Geometry check sheet. Reference: the model listing, model coordinates, mm. A direction names the side the tool comes from. Give positions to 0.01 mm unless a question says otherwise; leave off trailing zeros. Loops run counter-clockwise (first coordinate to the right, second up) from the corner with the lowest first, then second, coordinate; pieces in that order, holes last. Notation, with made-up numbers: (-22, 7) -> (-5, 7) arc R23 cw to (-5, 43) -> close; hole circle Ø9 at (26.5, 78). An arc over 180 degrees is marked (long way). Write item = value, one per line.
```python
from build123d import *

# Parameters (mm, degrees)
SKETCH1_W                                  = 120.9294
SKETCH1_H                                  = 116.1796
SKETCH1_R                                  = 10.5
SKETCH1_W_2                                = 11.906
SKETCH1_H_2                                = 30.0122
SKETCH1_W_3                                = 76.19975
SKETCH1_H_3                                = 95.2627
BOSS_EXTRUDE1_DEPTH                        = 4
SKETCH2_W                                  = 116.1796
SKETCH2_H                                  = 120.9294
SKETCH2_W_2                                = 102.459137156
SKETCH2_H_2                                = 106.648
BOSS_EXTRUDE2_DEPTH                        = 4.75
CUT_EXTRUDE1_DEPTH                         = 1.25
SKETCH6_W                                  = 25.4
SKETCH6_H                                  = 2.0635
SKETCH6_W_2                                = 1.783031422
SKETCH6_H_2                                = 25.4
CUT_EXTRUDE2_DEPTH                         = 2
CUT_EXTRUDE3_DEPTH                         = 10.16
SKETCH8_R                                  = 1.3
CUT_EXTRUDE4_DEPTH                         = 4
MIRROR1_AT_THE_SECOND_PLANE_COPY_1_SKETC_R = 1.3
MIRROR1_AT_THE_SECOND_PLANE_COPY_1_DEPTH   = 4
FILLET1_R                                  = 5
CHAMFER1_SIZE                              = 4


with BuildPart() as part:
    # Sketch1 → Boss-Extrude1 (new body)
    with BuildSketch(Plane(origin=(0, 0, 0), x_dir=(0, 1, 0), z_dir=(0, 0, 1))):
        Rectangle(SKETCH1_W, SKETCH1_H)
        with Locations(Location((39.3375, 10.8746, 0), (0, 0, 270))):
            Circle(SKETCH1_R, mode=Mode.SUBTRACT)
        with Locations((39.2905, -23.9125)):
            Rectangle(SKETCH1_W_2, SKETCH1_H_2, mode=Mode.SUBTRACT)
        with Locations((-11.906375, 0)):
            Rectangle(SKETCH1_W_3, SKETCH1_H_3, mode=Mode.SUBTRACT)
    extrude(amount=BOSS_EXTRUDE1_DEPTH)

    # Sketch2 → Boss-Extrude2 (add)
    with BuildSketch(Plane(origin=(0, 0, 0), x_dir=(-1, 0, 0), z_dir=(0, 0, -1))):
        Rectangle(SKETCH2_W, SKETCH2_H)
        Rectangle(SKETCH2_W_2, SKETCH2_H_2, mode=Mode.SUBTRACT)
    extrude(amount=BOSS_EXTRUDE2_DEPTH)

    # Sketch4 → Cut-Extrude1 (cut)
    with BuildSketch(Plane(origin=(0, 0, -4.75), x_dir=(-1, 0, 0), z_dir=(0, 0, -1))):
        Polygon((-50.0126, -52.3875), (-21, -52.3875), (-16, -57.3875), (16, -57.3875), (21, -52.3875), (50.0126, -52.3875), (50.0126, -21), (55.0126, -16), (55.0126, 16), (50.0126, 21), (50.0126, 52.3875), (21, 52.3875), (16, 57.3875), (-16, 57.3875), (-21, 52.3875), (-50.0126, 52.3875), (-50.0126, 21), (-55.0126, 16), (-55.0126, -16), (-50.0126, -21), align=None)
    extrude(amount=-CUT_EXTRUDE1_DEPTH, mode=Mode.SUBTRACT)

    # Sketch6 → Cut-Extrude2 (cut)
    with BuildSketch(Plane(origin=(0, 0, -3.5), x_dir=(1, 0, 0), z_dir=(0, 0, -1))):
        with Locations((0, 55.35575)):
            Rectangle(SKETCH6_W, SKETCH6_H)
        with Locations((0, -55.35575)):
            Rectangle(SKETCH6_W, SKETCH6_H)
        with Locations((-53.121084289, 0)):
            Rectangle(SKETCH6_W_2, SKETCH6_H_2)
        with Locations((53.121084289, 0)):
            Rectangle(SKETCH6_W_2, SKETCH6_H_2)
    extrude(amount=-CUT_EXTRUDE2_DEPTH, mode=Mode.SUBTRACT)

    # Sketch7 → Cut-Extrude3 (cut)
    with BuildSketch(Plane(origin=(-58.0898, 0, 0), x_dir=(0, -1, 0), z_dir=(-1, 0, 0))):
        with BuildLine():
            Line((-44.8211, 1.2342), (-34.9603, 1.2342))
            ThreePointArc((-34.9603, 1.2342), (-33.164248776, 0.490251224), (-32.4203, -1.3058))
            Line((-32.4203, -1.3058), (-32.4203, -5.3754))
            ThreePointArc((-32.4203, -5.3754), (-33.164248776, -7.171451224), (-34.9603, -7.9154))
            Line((-34.9603, -7.9154), (-44.8211, -7.9154))
            ThreePointArc((-44.8211, -7.9154), (-46.617151224, -7.171451224), (-47.3611, -5.3754))
            Line((-47.3611, -5.3754), (-47.3611, -1.3058))
            ThreePointArc((-47.3611, -1.3058), (-46.617151224, 0.490251224), (-44.8211, 1.2342))
        make_face()
    extrude(amount=-CUT_EXTRUDE3_DEPTH, mode=Mode.SUBTRACT)

    # Sketch8 → Cut-Extrude4 (cut)
    with BuildSketch(Plane(origin=(0, 0, -4.75), x_dir=(1, 0, 0), z_dir=(0, 0, -1))):
        with Locations(Location((-54.0258, 56.4007, 0), (0, 0, 180))):
            Circle(SKETCH8_R)
    cut_extrude4 = extrude(amount=-CUT_EXTRUDE4_DEPTH, mode=Mode.SUBTRACT)

    # Mirror1: Cut-Extrude4 across plane
    add(cut_extrude4.mirror(Plane(origin=(0, 0, 0), x_dir=(0, 0, 1), z_dir=(1, 0, 0))), mode=Mode.SUBTRACT)

    # Mirror1 at the second plane: Cut-Extrude4 across plane
    add(cut_extrude4.mirror(Plane.ZX), mode=Mode.SUBTRACT)

    # Mirror1 at the second plane copy 1 sketc → Mirror1 at the second plane copy 1 (cut)
    with BuildSketch(Plane(origin=(0, 0, -4.75), x_dir=(-1, 0, 0), z_dir=(0, 0, -1))):
        with Locations(Location((-54.0258, 56.4007, 0), (0, 0, 180))):
            Circle(MIRROR1_AT_THE_SECOND_PLANE_COPY_1_SKETC_R)
    extrude(amount=-MIRROR1_AT_THE_SECOND_PLANE_COPY_1_DEPTH, mode=Mode.SUBTRACT)

    # Fillet1
    fillet1_edges = [part.edges().sort_by_distance(p)[0] for p in [
        (58.0898, 60.4647, -0.375),
        (58.0898, -60.4647, -0.375),
        (-58.0898, -60.4647, -0.375),
        (-58.0898, 60.4647, -0.375),
    ]]
    fillet(fillet1_edges, radius=FILLET1_R)

    # Chamfer1
    # the kernel refuses this chamfer: 4 mm, written as the material it takes off along each edge
    with BuildSketch(Plane(origin=(-53.0898, -60.4647, 4), x_dir=(0, 0.9996219169112968, 0.027495876610586296), z_dir=(1, 0, 0)), Plane(origin=(53.0898, 60.4647, 4), x_dir=(0, -0.9996219169112968, 0.027495876610586296), z_dir=(-1, 0, 0))) as chamfer1_piece_1:
        Polygon((CHAMFER1_SIZE * 0.999621916911, -CHAMFER1_SIZE * 0.0274958766106), (-CHAMFER1_SIZE * 0.0274958766106, -CHAMFER1_SIZE * 0.999621916911), (0, 0), align=None)
    extrude(amount=106.1796, mode=Mode.SUBTRACT)
    with BuildSketch(Plane(origin=(58.0898, -55.4647, 4), x_dir=(0.02749587661058563, 0, -0.9996219169112968), z_dir=(0, 1, 0))) as chamfer1_piece_2:
        Polygon((CHAMFER1_SIZE * 0.999621916911, CHAMFER1_SIZE * 0.0274958766106), (-CHAMFER1_SIZE * 0.0274958766106, CHAMFER1_SIZE * 0.999621916911), (0, 0), align=None)
    extrude(amount=110.9294, mode=Mode.SUBTRACT)
    with BuildSketch(Plane(origin=(-58.0898, 55.4647, 4), x_dir=(0.9996219169112968, 0, 0.027495876610586296), z_dir=(0, -1, 0))) as chamfer1_piece_3:
        Polygon((CHAMFER1_SIZE * 0.999621916911, -CHAMFER1_SIZE * 0.0274958766106), (-CHAMFER1_SIZE * 0.0274958766106, -CHAMFER1_SIZE * 0.999621916911), (0, 0), align=None)
    extrude(amount=110.9294, mode=Mode.SUBTRACT)
    with BuildSketch(Plane(origin=(53.0898, 55.4647, 4), x_dir=(1, 0, 0), z_dir=(0, -1, 0))) as chamfer1_piece_4:
        Polygon((5 - CHAMFER1_SIZE, 0), (5, -CHAMFER1_SIZE), (5, 0), align=None)
    revolve(axis=Axis((53.0898, 55.4647, 4), (0, 0, 1)), revolution_arc=90, mode=Mode.SUBTRACT)
    with BuildSketch(Plane(origin=(53.0898, -55.4647, 4), x_dir=(1, 0, 0), z_dir=(0, 1, 0))) as chamfer1_piece_5:
        Polygon((5 - CHAMFER1_SIZE, 0), (5, CHAMFER1_SIZE), (5, 0), align=None)
    revolve(axis=Axis((53.0898, -55.4647, 4), (0, 0, -1)), revolution_arc=90, mode=Mode.SUBTRACT)
    with BuildSketch(Plane(origin=(-53.0898, 55.4647, 4), x_dir=(0, 1, 0), z_dir=(1, 0, 0))) as chamfer1_piece_6:
        Polygon((5 - CHAMFER1_SIZE, 0), (5, -CHAMFER1_SIZE), (5, 0), align=None)
    revolve(axis=Axis((-53.0898, 55.4647, 4), (0, 0, 1)), revolution_arc=90, mode=Mode.SUBTRACT)
    with BuildSketch(Plane(origin=(-53.0898, -55.4647, 4), x_dir=(0, -1, 0), z_dir=(1, 0, 0))) as chamfer1_piece_7:
        Polygon((5 - CHAMFER1_SIZE, 0), (5, CHAMFER1_SIZE), (5, 0), align=None)
    revolve(axis=Axis((-53.0898, -55.4647, 4), (0, 0, -1)), revolution_arc=90, mode=Mode.SUBTRACT)


solid = part.part
```
Item 1: Section check A-A, the plane y = 3.5. Record the cut outline in (x, z).
Answer:
outline = (-58.09, -4.75) -> (-55.01, -4.75) -> (-55.01, -3.5) -> (-54.01, -3.5) -> (-54.01, -1.5) -> (-52.23, -1.5) -> (-52.23, -3.5) -> (-51.23, -3.5) -> (-51.23, 0) -> (-47.63, 0) -> (-47.63, 4) -> (-54.09, 4) -> (-58.09, 0) -> close; (47.63, 0) -> (51.23, 0) -> (51.23, -3.5) -> (52.23, -3.5) -> (52.23, -1.5) -> (54.01, -1.5) -> (54.01, -3.5) -> (55.01, -3.5) -> (55.01, -4.75) -> (58.09, -4.75) -> (58.09, 0) -> (54.09, 4) -> (47.63, 4) -> close
Item 2: Section check B-B, the plane x = -24. Record the cut outline in (y, z), plus the area to 3 significant figures.
Answer:
outline = (-60.46, -4.75) -> (-53.32, -4.75) -> (-53.32, 0) -> (-50.01, 0) -> (-50.01, 4) -> (-56.46, 4) -> (-60.46, 0) -> close; (26.19, 0) -> (53.32, 0) -> (53.32, -4.75) -> (60.46, -4.75) -> (60.46, 0) -> (56.46, 4) -> (26.19, 4) -> close
area = 231 mm^2
Item 3: Section check D-D, the plane y = -40.5. Record the cut outline in (x, z).
Answer:
outline = (-58.09, -4.75) -> (-51.23, -4.75) -> (-51.23, 0) -> (-47.63, 0) -> (-47.63, 4) -> (-54.09, 4) -> (-58.09, 0) -> close; (47.63, 0) -> (51.23, 0) -> (51.23, -4.75) -> (58.09, -4.75) -> (58.09, 0) -> (54.09, 4) -> (47.63, 4) -> close
Item 4: Tool access check on faces 5 (the flat face through (-54, 56, -0.75)), 6 (the flat face through (1, -50.006, 2)), 7 (the flat face through (1, -60.465, -2)), 8 (the cylindrical face through (-53, 47, 0)). Record the directions out of +Z, -Z, +X, -X, +Y, -Y that give a thin tool (end or side, any length) a straight path to the whole face; none if there is none.
Answer:
face_5 = -Z
face_6 = +Z, -Z
face_7 = +Z, -Z, +X, -X, -Y
face_8 = -Z, -X
Item 5: Section check C-C, the plane x = 49. Record the cut outline in (y, z), plus the area to 3 significant figures.
Answer:
outline = (-60.46, -4.75) -> (-53.32, -4.75) -> (-53.32, 0) -> (53.32, 0) -> (53.32, -4.75) -> (60.46, -4.75) -> (60.46, 0) -> (56.46, 4) -> (-56.46, 4) -> (-60.46, 0) -> close
area = 536 mm^2
Item 6: Draft check along X on faces 1 (the cylindrical face through (53, 57.2, -2.8)), 2 (the cylindrical face through (56.664, -58.961, -2.408)), 3 (the flat face through (-0.743, -58.437, 2.028)), 4 (the flat face through (-47.631, -12, 2)). Enter one of: +X half, -X half, draft (parallel to the pull), parting line (faces both ways), or undercut.
Answer:
face_1 = undercut
face_2 = +X half
face_3 = draft
face_4 = undercut
Item 7: Gauge pin test, flat ends, axial feed: pin 1 (0.5 mm diameter, centred on x = -53.5, y = 5, fed in from -Z); pin 2 (1.6 mm diameter, centred on x = -54.03, y = -56.4, fed in from -Z); pin 3 (1.2 mm diameter, centred on x = 24, z = 2, fed in from +Y). Record the tip position at first contact, or that the pin passes through.
Answer:
pin_1 = -1.5
pin_2 = -0.75
pin_3 = 59.06
Item 8: Thickness scan on L1, parallel to X at y = -30.5, z = -3.75; L2, parallel to Y at x = 35.5, z = 1.25; L3, parallel to Y at x = -12.5, z = 2.5. Record the ranges inside material, lowest first. Write a range as [from, to].
Answer:
L1 = [-58.09, -51.23], [51.23, 58.09]
L2 = [-59.21, -50.01], [26.19, 33.34], [45.24, 59.21]
L3 = [-57.96, -50.01], [26.19, 28.96], [49.71, 57.96]
